Part model, mm, in its own coordinate system. Face numbers are marked on the shaded views. A direction names the side the tool comes from. Round coordinates to 2 decimals unless told otherwise and drop trailing zeros. Write each loop counter-clockwise with the first axis right and the second up, starting at its lowest first coordinate (ties: lowest second). Pieces come first, ordered by that corner, then holes. Notation, with made-up numbers: M 72.5,86 L 122.5,86 A22 ccw 122.5,119 Z; hole C 22.5,33 d3. An arc over 180 degrees is marked long. One line per question, with ' | ' between items. Start each with the question number.
1) Saw through at C-C (z = 15.5). List the corners of the cut face in (x, y).
2) Mould opens along Z. For the marked faces 3, 4 and 5 say: pulls with the +Z half, pulls with the -Z half, needs draft (parallel to the pull), parting line crosses it, or undercut.
3) Wall check: probe 1 along X at (y, z) = (-24, 18); probe 2 along X at (y, z) = (-33.5, -1); probe 3 along X at (y, z) = (-71, 12). Give the ranges that are in metal, low to high. Write a range as [from, to].
4) Saw through at A-A (y = -49.5). List the corners of the cut face in (x, z), plus the area to 3 significant figures.
5) Saw through at B-B (x = -14). List the corners of the cut face in (y, z), plus the area to 3 significant figures.
6) Drop flat-ended pins along their axis: pin 1 Ø5.5 at (x, y) = (-12.5, -106) entering from +Z; pin 2 Ø4 at (x, y) = (4, -74) entering from -Z; pin 3 Ø6.5 at (x, y) = (6, -56.5) entering from +Z. Give the stop position or say it passes through.
7) Tool access for the marked faces 1 and 2: list every direction of +Z, -Z, +X, -X, +Y, -Y with a clear straight run to the whole face (end or side of a thin tool).
8) Saw through at D-D (z = 25.5). List the corners of the cut face in (x, y).
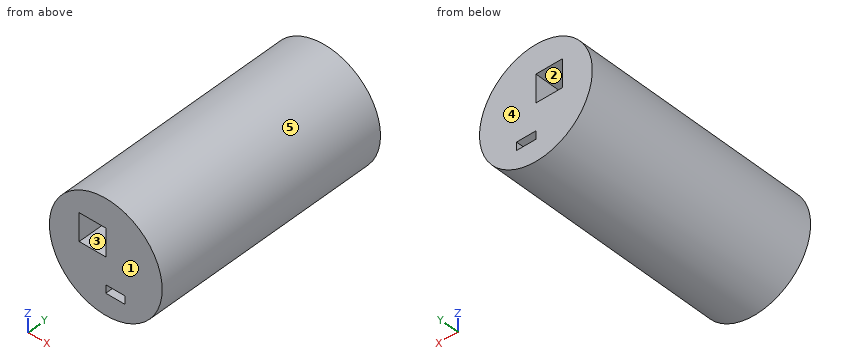
```python
from build123d import *

# Parameters (mm, degrees)
F0_R     = 37.264648
F0_W     = 12.802701
F0_H     = 5.376745
F0_W_2   = 17.537981
F0_H_2   = 18.3715
F1_DEPTH = 159.043342


with BuildPart() as f1:
    # F0 (on Front) → F1 (new body)
    with BuildSketch(Plane.XZ):
        Circle(F0_R)
        with Locations((6.40135, -20.412508)):
            Rectangle(F0_W, F0_H, mode=Mode.SUBTRACT)
        with Locations((-8.76899, 9.18575)):
            Rectangle(F0_W_2, F0_H_2, mode=Mode.SUBTRACT)
    extrude(amount=F1_DEPTH)


solid = f1.part
```
Answer key:
1) outline: M -33.89,-159.04 L -17.54,-159.04 L -17.54,0 L -33.89,0 Z; M 0,-159.04 L 33.89,-159.04 L 33.89,0 L 0,0 Z
2) face 3: undercut | face 4: needs draft | face 5: parting line crosses it
3) probe 1: x = [-32.63, -17.54], [0, 32.63] | probe 2: x = [-37.25, 37.25] | probe 3: x = [-35.28, -17.54], [0, 35.28]
4) outline: C 0,0 d74.53; hole M -17.54,0 L 0,0 L 0,18.37 L -17.54,18.37 Z; hole M 0,-23.1 L 12.8,-23.1 L 12.8,-17.72 L 0,-17.72 Z | area: 3,970 mm2
5) outline: M -159.04,-34.53 L 0,-34.53 L 0,0 L -159.04,0 Z; M -159.04,18.37 L 0,18.37 L 0,34.53 L -159.04,34.53 Z | area: 8,060 mm2
6) pin 1: stops at z = 35.97 | pin 2: stops at z = -37.21 | pin 3: stops at z = 37.16
7) face 1: +Z, -Z, +X, -X, -Y | face 2: +Y, -Y
8) outline: M -27.17,-159.04 L 27.17,-159.04 L 27.17,0 L -27.17,0 Z
